Build history of the part. All positions in model axes, mm. A direction names the side the tool comes from. Give positions to 0.01 mm unless a question says otherwise; leave off trailing zeros. Loops run counter-clockwise (first coordinate to the right, second up) from the corner with the lowest first, then second, coordinate; pieces in that order, holes last. Notation, with made-up numbers: (-14, 39) -> (24, 39) arc R13 cw to (24, 63) -> close; hole circle Ø6 at (-4.75, -39). An arc over 180 degrees is marked (long way). Answer as a JSON object with one key per item and string values. Group by question number.
from build123d import *

# Parameters (mm, degrees)
SKETCH4_R           = 50
SKETCH4_R_2         = 41.3
BOSS_EXTRUDE1_DEPTH = 50
SKETCH3_R           = 1.6
CUT_EXTRUDE1_DEPTH  = 10


with BuildPart() as part:
    # Sketch1 → Revolve1 (revolve)
    with BuildSketch(Plane.XY, mode=Mode.PRIVATE) as revolve1_sk:
        Polygon((39, 0), (39, 10), (55, 10), (55, -12), (41.5, -12), (41.5, 0), align=None)
    revolve(revolve1_sk.sketch.rotate(Axis((0, 83.520836207, 0), (0, -1, 0)), 90), axis=Axis((0, 83.520836207, 0), (0, -1, 0)))

    # Sketch4 → Boss-Extrude1 (add)
    with BuildSketch(Plane(origin=(0, 10, 0), x_dir=(1, 0, 0), z_dir=(0, 1, 0))):
        with Locations(Location((0, 0, 0), (0, 0, 270))):
            Circle(SKETCH4_R)
        with Locations(Location((0, 0, 0), (0, 0, 270))):
            Circle(SKETCH4_R_2, mode=Mode.SUBTRACT)
    extrude(amount=BOSS_EXTRUDE1_DEPTH)

    # Sketch3 → Cut-Extrude1 (cut)
    with BuildSketch(Plane.XZ.offset(12)):
        with Locations(Location((0, 48.25, 0), (0, 0, 270))):
            Circle(SKETCH3_R)
        with Locations(Location((48.25, 0, 0), (0, 0, 270))):
            Circle(SKETCH3_R)
        with Locations(Location((0, -48.25, 0), (0, 0, 270))):
            Circle(SKETCH3_R)
        with Locations(Location((-48.25, 0, 0), (0, 0, 270))):
            Circle(SKETCH3_R)
    extrude(amount=-CUT_EXTRUDE1_DEPTH, mode=Mode.SUBTRACT)


solid = part.part
(1) Pin check, flat tips, straight feed: pin 1 (1.6 mm diameter, centred on x = 48, z = 0, fed in from -Y); pin 2 (5 mm diameter, centred on y = 5.5, z = -17, fed in from +X); pin 3 (8 mm diameter, centred on x = -14.5, y = 36, fed in from +Z). Stop position of each tip, or through.
(2) Saw through at D-D on z = -17. List the corners of the cut face in (x, y), plus the area to 3 significant figures.
(3) 3-axis set-ups, long thin cutter, end or side, ignore diameter. For faces 1 (the cylindrical face through (-38.668, 5.07, -5.077)), 2 (the flat face through (-48, -2, 0)), 3 (the cylindrical face through (15.02, 34.65, 47.69)): which of +Z, -Z, +X, -X, +Y, -Y reach the whole face in a straight line?
(4) Saw through at C-C on y = 24. List the corners of the cut face in (x, z).
(5) Pull direction X, two halves, no side cores. Call faces 4 (the flat face through (49, 10, -12)), 5 (the cylindrical face through (12.41, 34.65, 39.39)), 6 (the cylindrical face through (49.6, -7.07, -0.86)), 7 (the cylindrical face through (48.794, -1.154, 25.379)): pulls with the +X half, pulls with the -X half, needs draft (parallel to the pull), parting line crosses it, or undercut.
(6) Probe line 1 along X through (y, z) = (-9, 0); line 2 along Y through (x, z) = (-30, -45); line 3 along X through (y, z) = (-7.5, -48.25). List the from-to ranges inside material, lowest first. Write a range as [from, to].
(7) Saw through at A-A on z = 0. List the corners of the cut face in (x, y).
(8) Saw through at B-B on x = 0. List the corners of the cut face in (y, z), plus the area to 3 significant figures.
Calculated:
{
 "1": {"pin 1": "stops at y = -2", "pin 2": "stops at x = 53.05", "pin 3": "stops at z = 48.89"},
 "2": {"outline": "(-52.31, -12) -> (-37.86, -12) -> (-37.86, 0) -> (-35.1, 0) -> (-35.1, 10) -> (-37.64, 10) -> (-37.64, 60) -> (-47.02, 60) -> (-47.02, 10) -> (-52.31, 10) -> close; (35.1, 0) -> (37.86, 0) -> (37.86, -12) -> (52.31, -12) -> (52.31, 10) -> (47.02, 10) -> (47.02, 60) -> (37.64, 60) -> (37.64, 10) -> (35.1, 10) -> close", "area": "1,630 mm^2"},
 "3": {"face 1": "+Y, -Y", "face 2": "-Y", "face 3": "+Y"},
 "4": {"outline": "circle Ø100 at (0, 0); hole circle Ø82.6 at (0, 0)"},
 "5": {"face 4": "needs draft", "face 5": "undercut", "face 6": "undercut", "face 7": "parting line crosses it"},
 "6": {"line 1": "x = [-55, -49.85], [-46.65, -41.5], [41.5, 46.65], [49.85, 55]", "line 2": "y = [-12, 10]", "line 3": "x = [-26.4, -1.6], [1.6, 26.4]"},
 "7": {"outline": "(-55, -12) -> (-49.85, -12) -> (-49.85, -2) -> (-46.65, -2) -> (-46.65, -12) -> (-41.5, -12) -> (-41.5, 0) -> (-39, 0) -> (-39, 10) -> (-41.3, 10) -> (-41.3, 60) -> (-50, 60) -> (-50, 10) -> (-55, 10) -> close; (39, 0) -> (41.5, 0) -> (41.5, -12) -> (46.65, -12) -> (46.65, -2) -> (49.85, -2) -> (49.85, -12) -> (55, -12) -> (55, 10) -> (50, 10) -> (50, 60) -> (41.3, 60) -> (41.3, 10) -> (39, 10) -> close"},
 "8": {"outline": "(-12, -55) -> (10, -55) -> (10, -50) -> (60, -50) -> (60, -41.3) -> (10, -41.3) -> (10, -39) -> (0, -39) -> (0, -41.5) -> (-12, -41.5) -> (-12, -46.65) -> (-2, -46.65) -> (-2, -49.85) -> (-12, -49.85) -> close; (-12, 41.5) -> (0, 41.5) -> (0, 39) -> (10, 39) -> (10, 41.3) -> (60, 41.3) -> (60, 50) -> (10, 50) -> (10, 55) -> (-12, 55) -> (-12, 49.85) -> (-2, 49.85) -> (-2, 46.65) -> (-12, 46.65) -> close", "area": "1,450 mm^2"}
}
